Read the model definition and answer for the solid it produces. Units are mm, in the model's axes. A direction names the side the tool comes from. Give positions to 0.01 mm unless a question says otherwise; leave off trailing zeros. Order: outer loops, then holes, each group sorted by start corner. A loop starts at its lowest first (then second) coordinate and runs counter-clockwise, first axis right, second up. Notation, with made-up numbers: (60.5, 14) - (77.5, 14) arc R3 ccw to (77.5, 18) - close; hole circle Ø10 at (-15.75, 73). An arc over 180 degrees is marked (long way). Write each question's results on one line, items separated by ' | '.
Autodesk Inventor part; units mm, degrees
ref_plane "YZ Plane" through (0, 0, 0) normal (1, 0, 0) x (0, 1, 0)
ref_plane "XZ Plane" through (0, 0, 0) normal (0, 1, 0) x (-1, 0, 0)
ref_plane "XY Plane" through (0, 0, 0) normal (0, 0, 1) x (1, 0, 0)
sketch "Skizze1" plane through (0, 0, 0) normal (0, 0, 1) x (1, 0, 0)
  line L0 (-68.016, 1.808) -> (67.584, 1.808)
  line L1 (67.584, 1.808) -> (67.584, -2.192)
  line L2 (67.584, -2.192) -> (-68.016, -2.192)
  line L3 (-68.016, -2.192) -> (-68.016, 1.808)
  line L4 (-68.016, 1.808) -> (67.584, -2.192) construction
  line L5 (67.584, 1.808) -> (-68.016, -2.192) construction
  point P0 (0, 0)
  point P1 (-0.216, -0.192)
  point P2 (-0.216, -0.192)
  dimension "d0" = 135.6
  dimension "d1" = 4
extrude "Extrusion1" add sketch "Skizze1" along normal mid plane 3.25
ref_plane "Arbeitsebene1" through (-68.016, -0.192, 1.625) normal (0, -1, 0) x (1, 0, 0)
sketch "Skizze2" plane through (-68.016, -0.192, 1.625) normal (0, -1, 0) x (1, 0, 0)
  line L0 (0, -3.25) -> (0, 0)
  line L1 (0, -3.25) -> (135.6, -3.25)
  line L2 (0, 0) -> (2.85, 0)
  line L3 (2.85, 0) -> (2.85, -3.25)
  line L4 (2.85, -3.25) -> (0, -3.25)
  line L5 (0, -3.25) -> (0, 0)
  line L6 (0, 0) -> (0, 1.75)
  line L7 (0, 1.75) -> (2.85, 0)
  line L8 (135.6, -3.25) -> (135.6, 0)
  line L9 (135.6, 0) -> (132.75, 0)
  line L10 (132.75, 0) -> (132.75, -3.25)
  line L11 (132.75, -3.25) -> (135.6, -3.25)
  line L12 (135.6, -3.25) -> (135.6, 0)
  line L13 (135.6, 0) -> (135.6, 1.75)
  line L14 (135.6, 1.75) -> (132.75, 0)
  point P0 (68.016, -1.625)
  dimension "d4" = 2.85
  dimension "d5" = 1.75
  dimension "d6" = 2.85
extrude "Extrusion2" add sketch "Skizze2" along normal mid plane 19.7
sketch "Skizze7" plane through (0, 0, 1.625) normal (0, 0, 1) x (1, 0, 0)
  line L0 (-65.166, 9.658) -> (-65.166, 1.808)
  line L1 (-65.166, 1.808) -> (-55.166, 1.808)
  line L2 (64.734, 1.808) -> (-65.166, 1.808)
  line L3 (64.734, -2.192) -> (-65.166, -2.192)
  line L4 (64.734, -2.192) -> (54.734, -2.192)
  line L5 (-55.166, 1.808) -> (54.734, 1.808)
  line L6 (54.734, 1.808) -> (54.734, -2.192)
  line L7 (54.734, -2.192) -> (-55.166, -2.192)
  line L8 (-55.166, -2.192) -> (-55.166, 1.808)
  point P0 (0, 0)
  dimension "d27" = 10
  dimension "d28" = 10
extrude "Extrusion7" add sketch "Skizze7" along normal blind 26.5
sketch "Skizze8" plane through (0, 0, 1.625) normal (0, 0, 1) x (1, 0, 0)
  line L0 (-65.166, 1.808) -> (-50.166, 1.808)
  line L1 (-65.166, 1.808) -> (64.734, 1.808)
  line L2 (64.734, -2.192) -> (-65.166, -2.192)
  line L3 (64.734, -2.192) -> (49.734, -2.192)
  line L4 (-50.166, 1.808) -> (49.734, 1.808)
  line L5 (49.734, 1.808) -> (49.734, -2.192)
  line L6 (49.734, -2.192) -> (-50.166, -2.192)
  line L7 (-50.166, -2.192) -> (-50.166, 1.808)
  point P0 (0, 0)
  dimension "d31" = 15
  dimension "d32" = 15
extrude "Extrusion8" cut sketch "Skizze8" along normal blind 21.5
ref_plane "Arbeitsebene2" through (-0.216, -10.042, -1.625) normal (-1, 0, 0) x (0, 0, 1)
sketch "Skizze9" plane through (-0.216, -10.042, -1.625) normal (-1, 0, 0) x (0, 0, 1)
  line L0 (24.75, 11.85) -> (29.75, 11.85)
  line L1 (29.75, 11.85) -> (29.75, 7.85)
  line L2 (29.75, 7.85) -> (24.75, 7.85)
  line L3 (24.75, 7.85) -> (24.75, 11.85)
  point P0 (1.625, 10.042)
extrude "Extrusion9" cut sketch "Skizze9" along normal mid plane 14
sketch "Skizze17" plane through (-0.216, -10.042, -1.625) normal (-1, 0, 0) x (0, 0, 1)
  line L0 (24.75, 11.85) -> (24.75, 28.85)
  line L1 (62.75, -9.15) -> (62.75, 28.85)
  line L2 (24.75, 28.85) -> (62.75, 28.85)
  line L3 (62.75, 28.85) -> (62.75, -9.15)
  line L4 (62.75, -9.15) -> (24.75, -9.15)
  line L5 (24.75, -9.15) -> (24.75, 28.85)
  circle A0 centre (43.75, 9.85) radius 14
  point P0 (1.625, 10.042)
extrude "Extrusion19" add sketch "Skizze17" along normal mid plane 21
sketch "Skizze19" plane through (-0.216, -10.042, -1.625) normal (-1, 0, 0) x (0, 0, 1)
  line L0 (24.75, 28.85) -> (24.75, 11.85)
  line L1 (24.75, -9.15) -> (62.75, -9.15)
  line L2 (24.75, 28.85) -> (62.75, 28.85)
  line L3 (62.75, 28.85) -> (62.75, -9.15)
  line L4 (62.75, -9.15) -> (24.75, -9.15)
  line L5 (24.75, -9.15) -> (24.75, 28.85)
  point P0 (1.625, 10.042)
  point P1 (24.75, 11.85)
extrude "Extrusion20" cut sketch "Skizze19" along normal mid plane 16
sketch "Skizze20" plane through (10.284, -19.192, 61.125) normal (0, 0, 1) x (1, 0, 0)
  line L0 (0, 38) -> (0, 0)
  line L1 (0, 38) -> (-21, 38)
  line L2 (-21, 38) -> (-21, 0)
  line L3 (-21, 0) -> (0, 0)
  line L4 (0, 0) -> (0, 38)
  point P0 (-10.284, 19.192)
extrude "Extrusion21" add sketch "Skizze20" along normal blind 2.5
sketch "Skizze21" plane through (7.784, -19.192, 23.125) normal (0, -1, 0) x (1, 0, 0)
  line L0 (-18.5, 5) -> (-18.5, 33)
  line L1 (2.5, 40.5) -> (-18.5, 40.5)
  line L2 (-18.5, 40.5) -> (-18.5, 19)
  line L3 (-18.5, 19) -> (2.5, 19)
  line L4 (2.5, 19) -> (2.5, 40.5)
  point P0 (-7.784, -23.125)
extrude "Extrusion22" add sketch "Skizze21" along normal blind 2.5
sketch "Skizze22" plane through (0, 0, 23.125) normal (0, 0, -1) x (-1, 0, 0)
  line L0 (-54.734, 1.808) -> (-10.284, 1.808)
  line L1 (-10.284, 1.808) -> (-7.784, 1.808)
  line L2 (-7.784, 18.808) -> (-7.784, -19.192)
  line L3 (-10.284, 1.808) -> (-7.784, 1.808) construction
  line L4 (-10.284, -2.192) -> (-54.734, -2.192)
  line L5 (-7.784, 1.808) -> (-10.784, 1.808)
  line L6 (-10.784, 1.808) -> (-10.784, -2.192)
  line L7 (-10.784, -2.192) -> (-7.784, -2.192)
  line L8 (-7.784, -2.192) -> (-7.784, 1.808)
  line L9 (10.716, 18.808) -> (10.716, -21.692)
  line L10 (10.716, -2.192) -> (8.216, -2.192)
  line L11 (8.216, -2.192) -> (11.216, -2.192)
  line L12 (11.216, -2.192) -> (11.216, 1.808)
  line L13 (11.216, 1.808) -> (8.216, 1.808)
  line L14 (8.216, 1.808) -> (8.216, -2.192)
  point P0 (0, 0)
  dimension "d79" = 2.5
  dimension "d80" = 0
  dimension "d81" = 3
  dimension "d82" = 2.5
  dimension "d83" = 3
extrude "Extrusion23" add sketch "Skizze22" along normal up to surface (24.75 mm away)
properties part number "2024_09_24_Holder_Power_sensor"
(1) Consider probe 1 along X at (y, z) = (-14, 31); probe 2 along Y at (x, z) = (-51, 3); probe 3 along Z at (x, y) = (-47, 0) (3 decimals). Determine where each line is inside the solid, lowest interval first. Write a range as [from, to].
Conclusion:
probe 1: [-10.72, -8.22], [7.78, 10.28] | probe 2: [-2.19, 1.81] | probe 3: [-1.625, 1.625], [23.125, 28.125]
(2) Each of these flat-tipped pins is pushed along its axis until it touches: pin 1 (2 mm diameter, centred on x = 49.5, z = 21, fed in from +Y); pin 2 (1.5 mm diameter, centred on y = -4, z = 23, fed in from -X); pin 3 (1.2 mm diameter, centred on y = -1, z = 10, fed in from +X). Where does it stop, or does it pass through?
Conclusion:
pin 1: y = 1.81 | pin 2: x = -10.72 | pin 3: x = 54.73
(3) Section B-B (z = 25.5) is taken. Give the vertices of the cut face in (x, y).
Conclusion:
outline: (-55.17, -2.19) - (-10.72, -2.19) - (-10.72, -19.19) - (-8.22, -19.19) - (-8.22, 18.81) - (-10.72, 18.81) - (-10.72, 1.81) - (-55.17, 1.81) - close; (7.78, -19.19) - (10.28, -19.19) - (10.28, -2.19) - (54.73, -2.19) - (54.73, 1.81) - (10.28, 1.81) - (10.28, 18.81) - (7.78, 18.81) - close
(4) For faces 1 (the face through (-33, 0, 28.125)), 2 (the face through (-65.166, -6, 0)), 3 (the face through (60, 0, 1.625)), determine the directions among +Z, -Z, +X, -X, +Y, -Y from which every point of the face is accessible in a straight line to the end or side of a thin tool.
Conclusion:
face 1: +Z, -X, +Y, -Y | face 2: +Z, -Z, -Y | face 3: +Z, +Y, -Y
(5) The mould has two halves that part along Z. Classify faces 4 (the face through (-67, 9.658, 0)), 5 (the face through (-9.45, -0.81, 28.14)), 6 (the face through (9, 10, 23.125)), 7 (the face through (30, 0, 1.625)): pulls with the +Z half, pulls with the -Z half, needs draft (parallel to the pull), parting line crosses it, or undercut.
Conclusion:
face 4: needs draft | face 5: undercut | face 6: pulls with the -Z half | face 7: undercut
(6) Section C-C (z = 48) is taken. Give the vertices of the cut face in (x, y).
Conclusion:
outline: (-10.72, -21.69) - (10.28, -21.69) - (10.28, -12.9) - (7.78, -12.9) - (7.78, -19.19) - (-8.22, -19.19) - (-8.22, -12.9) - (-10.72, -12.9) - close; (-10.72, 12.52) - (-8.22, 12.52) - (-8.22, 18.81) - (-10.72, 18.81) - close; (7.78, 12.52) - (10.28, 12.52) - (10.28, 18.81) - (7.78, 18.81) - close
(7) Section D-D (z = 9) is taken. Give the vertices of the cut face in (x, y), plus the area to 3 significant figures.
Conclusion:
outline: (-55.17, -2.19) - (-50.17, -2.19) - (-50.17, 1.81) - (-55.17, 1.81) - close; (-11.22, -2.19) - (-8.22, -2.19) - (-8.22, 1.81) - (-11.22, 1.81) - close; (7.78, -2.19) - (10.78, -2.19) - (10.78, 1.81) - (7.78, 1.81) - close; (49.73, -2.19) - (54.73, -2.19) - (54.73, 1.81) - (49.73, 1.81) - close | area: 64.0 mm^2
(8) Section A-A (x = 1.5) is taken. Give the vertices of the cut face in (y, z) (3 decimals).
Conclusion:
outline: (-21.692, 42.125) - (-19.192, 42.125) - (-19.192, 61.125) - (18.808, 61.125) - (18.808, 63.625) - (-21.692, 63.625) - close; (-2.192, -1.625) - (1.808, -1.625) - (1.808, 1.625) - (-2.192, 1.625) - close
